from build123d import *

# Parameters (mm, degrees)
F1_DEPTH  = 17
F2_W      = 12.8
F2_H      = 16.8
F3_DEPTH  = 16.8
F5_DEPTH  = 5
F11_W     = 3.8
F11_H     = 2
F12_DEPTH = 1


with BuildPart() as f1:
    # F0 (on Front) → F1 (new body)
    with BuildSketch(Plane.XZ):
        Polygon((0, 20), (0, 0), (20, 0), (20, 3.2), (3.2, 20), align=None)
    extrude(amount=F1_DEPTH)

    # F2 (on face) → F3 (cut)
    with BuildSketch(Plane.YZ.offset(20)):
        with Locations((-8.5, 11.6)):
            Rectangle(F2_W, F2_H)
    extrude(amount=-F3_DEPTH, mode=Mode.SUBTRACT)


with BuildPart() as f5:
    # F4 (on face) → F5 (new body)
    with BuildSketch(Plane(origin=(0, 0, 0), x_dir=(0, -1, 0), z_dir=(-1, 0, 0))):
        with BuildLine():
            ThreePointArc((5.25, 8.75), (8.5, 5.5), (11.75, 8.75))
            Line((11.75, 8.75), (11.75, 11.25))
            ThreePointArc((11.75, 11.25), (8.5, 14.5), (5.25, 11.25))
            Line((5.25, 11.25), (5.25, 8.75))
        make_face()
    extrude(amount=-F5_DEPTH)


with BuildPart() as f9_1:
    # F9: instance of F5
    add(f5.part.mirror(Plane(origin=(11.6, -2.1, 11.6), x_dir=(-0.7071067812, 0, -0.7071067812), z_dir=(0.7071067812, 0, -0.7071067812))))


with BuildPart() as f1_1:
    add(f1.part)

    # F10: cut F5, F9_1
    add(f5.part, mode=Mode.SUBTRACT)
    add(f9_1.part, mode=Mode.SUBTRACT)



with BuildPart() as f12:
    # F11 (on face) → F12 (new body)
    with BuildSketch(Plane(origin=(0, 0, 0), x_dir=(0, -1, 0), z_dir=(-1, 0, 0))):
        with Locations((8.5, 17.25)):
            Rectangle(F11_W, F11_H)
    extrude(amount=F12_DEPTH)


with BuildPart() as f12b:
    # F11 (on face) → F12, piece 2 (new body)
    with BuildSketch(Plane(origin=(0, 0, 0), x_dir=(0, -1, 0), z_dir=(-1, 0, 0))):
        with Locations((8.5, 2.75)):
            Rectangle(F11_W, F11_H)
    extrude(amount=F12_DEPTH)


with BuildPart() as f1_2:
    add(f1_1.part)

    add(f12.part)  # F13 merges F12

    add(f12b.part)  # F13 merges F12b
    # F13: F12, F12b across plane
    add(f12.part.mirror(Plane(origin=(11.6, -2.1, 11.6), x_dir=(-0.7071067812, 0, -0.7071067812), z_dir=(0.7071067812, 0, -0.7071067812))))
    add(f12b.part.mirror(Plane(origin=(11.6, -2.1, 11.6), x_dir=(-0.7071067812, 0, -0.7071067812), z_dir=(0.7071067812, 0, -0.7071067812))))


solid = f1_2.part
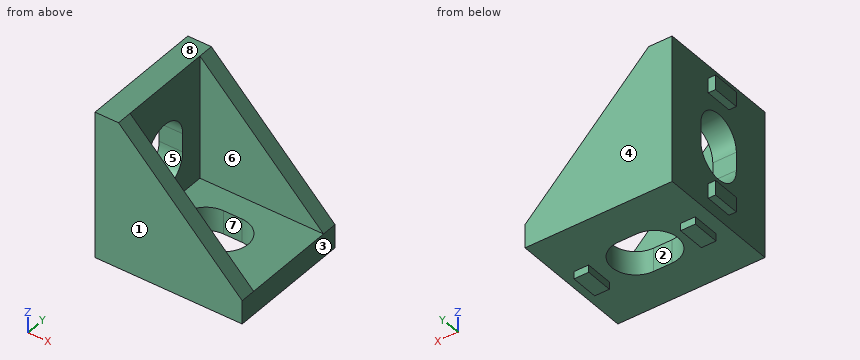
Input: part model. Units: mm. Frame: model coordinates. Face numbers are marked on the shaded views. A direction names the side the tool comes from. Round coordinates to 2 decimals unless told otherwise and drop trailing zeros. Order: outer loops, then holes, each group sorted by start corner. A loop starts at its lowest first (then second) coordinate and runs counter-clockwise, first axis right, second up. Notation, with made-up numbers: (-2, -6) - (31, -6) arc R8 ccw to (31, 2) - close; hole circle Ø11 at (45, -22). An arc over 180 degrees is marked (long way). Answer as a JSON object with one key per item and string values. Group by question number.
(1) Cut plane D-D (z = 18.75). Return loops of the section in (x, y), then the cut area to 4 significant figures.
(2) Cut plane C-C (y = -5.75). Return loops of the section in (x, z), then the cut area to 3 significant figures.
(3) Material intervals for probe 1 along Y at (x, z) = (6.25, 13.75); probe 2 along Z at (x, y) = (4, -10); probe 3 along Z at (x, y) = (0.25, -15.5), sorted ascending. Write a range as from..to.
(4) Cut plane A-A (x = 7.5). Return loops of the section in (y, z).
(5) Cut plane B-B (x = 1.25). Return loops of the section in (y, z), then the cut area to 3 significant figures.
(6) Draft query along Y for the marked faces 1, 2, 3 and 4. Return one class per face: released by +Y, released by -Y, zero draft, split by the parting line, or undercut.
(7) Pin query (flat end, axial travel): P1, Ø3, axis at x = 9, y = -6, coming from the -Z side; P2, Ø0.5, axis at x = -0.5, z = 3, coming from the +Y side; P3, Ø2, axis at x = 10, y = -12.5, coming from the +Z side. Return the tip coordinate at first contact, or that it passes through.
(8) Reachability of the marked faces 5, 6, 7 and 8 from +Z, -Z, +X, -X, +Y, -Y: full face, straight path, thin tool, end or side. Return the list, or none.
Here are the results:
{
 "1": {"outline": "(0, -17) - (4.45, -17) - (4.45, -14.9) - (3.2, -14.9) - (3.2, -2.1) - (4.45, -2.1) - (4.45, 0) - (0, 0) - close", "area": "59.65 mm^2"},
 "2": {"outline": "(0, 0) - (7.02, 0) - (7.02, 3.2) - (3.2, 3.2) - (3.2, 7.02) - (0, 7.02) - close; (0, 12.98) - (3.2, 12.98) - (3.2, 20) - (0, 20) - close; (12.98, 0) - (20, 0) - (20, 3.2) - (12.98, 3.2) - close", "area": "79.6 mm^2"},
 "3": {"probe 1": "y = -17..-14.9, -2.1..0", "probe 2": "z = 0..3.2", "probe 3": "z = 0..20"},
 "4": {"outline": "(-17, 0) - (-11.5, 0) - (-11.5, 3.2) - (-14.9, 3.2) - (-14.9, 15.7) - (-17, 15.7) - close; (-5.5, 0) - (0, 0) - (0, 15.7) - (-2.1, 15.7) - (-2.1, 3.2) - (-5.5, 3.2) - close"},
 "5": {"outline": "(-17, 0) - (0, 0) - (0, 20) - (-17, 20) - close; hole (-11.75, 8.75) arc R3.25 ccw to (-5.25, 8.75) - (-5.25, 11.25) arc R3.25 ccw to (-11.75, 11.25) - close", "area": "291 mm^2"},
 "6": {"face 1": "released by -Y", "face 2": "undercut", "face 3": "zero draft", "face 4": "released by +Y"},
 "7": {"P1": "stops at z = 0", "P2": "stops at y = -6.6", "P3": "stops at z = 3.2"},
 "8": {"face 5": "+X, -X", "face 6": "+Z, +X", "face 7": "+Z, -Z", "face 8": "+Z, +X, -X, +Y, -Y"}
}
